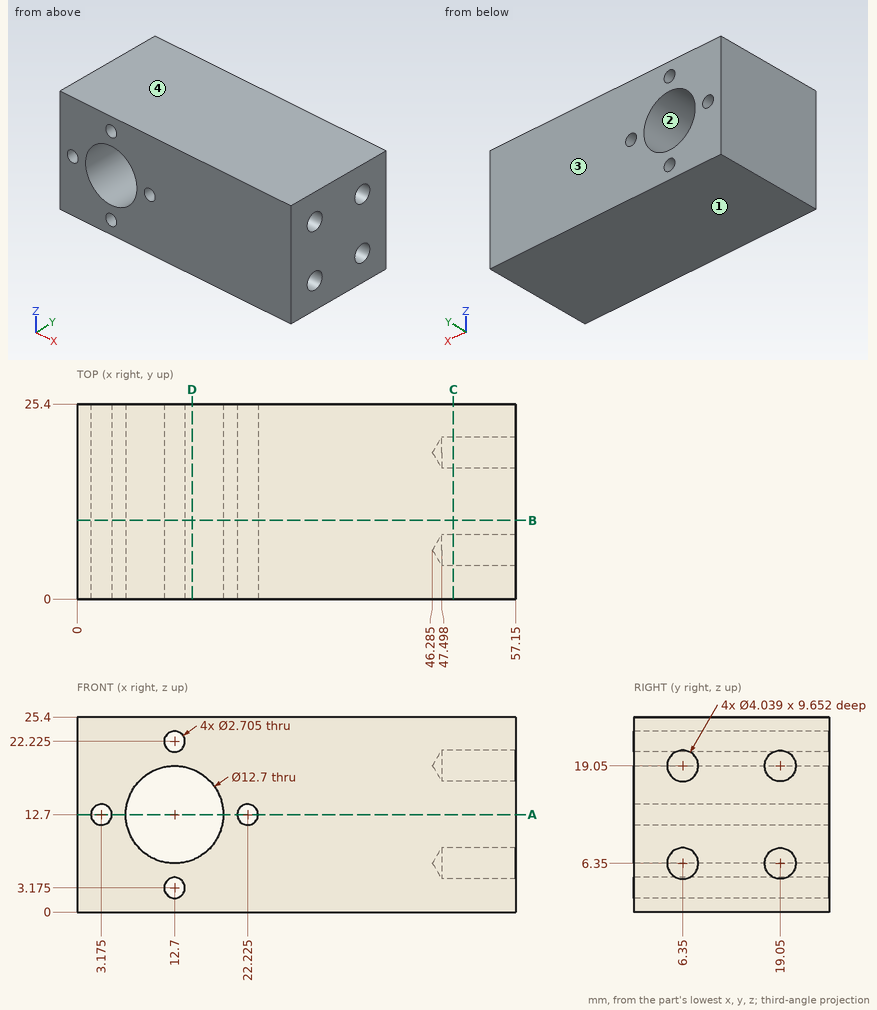
For this review, use the dimensioned drawing (mm, ordinates from the lowest corner) and the shaded views. Round coordinates to 2 decimals unless told otherwise and drop trailing zeros. Order: outer loops, then holes, each group sorted by start corner. A loop starts at its lowest first (then second) coordinate and runs counter-clockwise, first axis right, second up. Notation, with made-up numbers: M 14,39.5 L 53,39.5 A32 ccw 53,71.5 Z; hole C 35,50.25 d11. An arc over 180 degrees is marked long. Write each question's results on one line, items separated by ' | '. Start each with the question number.
1. Add section B-B (y = 10.25). State how many separate pieces and enclosed holes the cut face has, then the cut area to 3 significant figures.
2. Clearance check with a flat-ended pin moving along its axis: pin 1 Ø2.5 at (y, z) = (6.35, 6.35) entering from +X (1 decimal). State where the tip first meets the part, or that it passes through.
3. Add section A-A (z = 12.7). State the section outline as (x, y) points.
4. Add section D-D (x = 15). State the section outline as (y, z) points.
5. Draft analysis for pull direction Z (two halves, no side actions). For the marked faces 1, 2, 3 and 4, state which applies: pulls with the +Z half, pulls with the -Z half, needs draft (parallel to the pull), parting line crosses it, or undercut.
6. To check wall thickness, follow L1, parallel to Z at x = 49, y = 6.5; L2, parallel to Y at x = 54.5, z = 19.05; L3, parallel to X at y = 11.5, z = 11.75. State the ranges of each line that lie inside material, in increasing order. Write a range as [from, to].
7. Add section C-C (x = 49). State the section outline as (y, z) points.
Output values:
1) separate pieces: 1 | enclosed holes: 5 | area: 1,300 mm^2
2) pin 1: x = 47
3) outline: M 0,0 L 1.82,0 L 1.82,25.4 L 0,25.4 Z; M 4.53,0 L 6.35,0 L 6.35,25.4 L 4.53,25.4 Z; M 19.05,0 L 20.87,0 L 20.87,25.4 L 19.05,25.4 Z; M 23.58,0 L 57.15,0 L 57.15,25.4 L 23.58,25.4 Z
4) outline: M 0,0 L 25.4,0 L 25.4,6.78 L 0,6.78 Z; M 0,18.62 L 25.4,18.62 L 25.4,25.4 L 0,25.4 Z
5) face 1: pulls with the -Z half | face 2: undercut | face 3: needs draft | face 4: pulls with the +Z half
6) L1: [0, 4.34], [8.36, 17.04], [21.06, 25.4] | L2: [0, 4.33], [8.37, 17.03], [21.07, 25.4] | L3: [0, 2.21], [4.14, 6.42], [18.98, 21.26], [23.19, 57.15]
7) outline: M 0,0 L 25.4,0 L 25.4,25.4 L 0,25.4 Z; hole C 6.35,6.35 d4.04; hole C 6.35,19.05 d4.04; hole C 19.05,6.35 d4.04; hole C 19.05,19.05 d4.04
